Read the model definition and answer for the solid it produces. Units are mm, in the model's axes. Face numbers are marked on the shaded views. Give positions to 0.01 mm unless a question says otherwise; leave off trailing zeros. Order: outer loops, then holes, each group sorted by start corner. A loop starts at its lowest first (then second) coordinate and runs counter-clockwise, first axis right, second up. Notation, with made-up numbers: (60, -40) - (106, -40) arc R14 ccw to (106, -28) - close; hole circle Ø2 at (-27.75, -14). An arc over 180 degrees is marked (long way). Write each question's results on one line, items separated by ' | '.
from build123d import *

# Parameters (mm, degrees)
SKETCH1_W             = 7
SKETCH1_H             = 12
BOSS_EXTRUDE1_DEPTH   = 5
SKETCH1_W_2           = 8.5
BOSS_EXTRUDE1_2_DEPTH = 5
SKETCH3_W             = 122.5
SKETCH3_H             = 12
BOSS_EXTRUDE2_DEPTH   = 3
SKETCH4_R             = 1.4
CUT_EXTRUDE1_DEPTH    = 3
FILLET1_R             = 3


with BuildPart() as part:
    # Sketch1 → Boss-Extrude1 (new body)
    with BuildSketch(Plane(origin=(0, 0, 0), x_dir=(0, 0, -1), z_dir=(1, 0, 0))):
        with Locations((-57, 0)):
            Rectangle(SKETCH1_W, SKETCH1_H)
    extrude(amount=BOSS_EXTRUDE1_DEPTH)



with BuildPart() as body_2:
    # Sketch1 → Boss-Extrude1 2 (new body)
    with BuildSketch(Plane(origin=(0, 0, 0), x_dir=(0, 0, -1), z_dir=(1, 0, 0))):
        with Locations((57.75, 0)):
            Rectangle(SKETCH1_W_2, SKETCH1_H)
    extrude(amount=BOSS_EXTRUDE1_2_DEPTH)


with BuildPart() as part_1:
    add(part.part)

    add(body_2.part)  # Boss-Extrude2 merges body 2
    # Sketch3 → Boss-Extrude2 (add)
    with BuildSketch(Plane(origin=(5, 0, 0), x_dir=(0, 0, -1), z_dir=(1, 0, 0))):
        with Locations((0.75, 0)):
            Rectangle(SKETCH3_W, SKETCH3_H)
    extrude(amount=BOSS_EXTRUDE2_DEPTH)

    # Sketch4 → Cut-Extrude1 (cut)
    with BuildSketch(Plane(origin=(8, 0, 0), x_dir=(0, 0, -1), z_dir=(1, 0, 0))):
        with BuildLine():
            Line((-19.25, 4.4), (-29.25, 4.4))
            ThreePointArc((-29.25, 4.4), (-30.65, 3), (-29.25, 1.6))
            Line((-29.25, 1.6), (-19.25, 1.6))
            ThreePointArc((-19.25, 1.6), (-20.65, 3), (-19.25, 4.4))
        make_face()
        with Locations((-19.25, 3)):
            Circle(SKETCH4_R)
        with BuildLine():
            Line((-9.25, 4.4), (-19.25, 4.4))
            ThreePointArc((-19.25, 4.4), (-18.260050506, 3.989949494), (-17.85, 3))
            ThreePointArc((-17.85, 3), (-18.260050506, 2.010050506), (-19.25, 1.6))
            Line((-19.25, 1.6), (-9.25, 1.6))
            ThreePointArc((-9.25, 1.6), (-7.85, 3), (-9.25, 4.4))
        make_face()
        with BuildLine():
            Line((-9.25, -1.6), (-19.250000006, -1.6))
            ThreePointArc((-19.250000006, -1.6), (-18.260050509, -2.010050504), (-17.85, -3))
            ThreePointArc((-17.85, -3), (-18.260050506, -3.989949494), (-19.25, -4.4))
            Line((-19.25, -4.4), (-9.25, -4.4))
            ThreePointArc((-9.25, -4.4), (-7.85, -3), (-9.25, -1.6))
        make_face()
        with Locations((-19.25, -3)):
            Circle(SKETCH4_R)
        with BuildLine():
            Line((-19.250000006, -1.6), (-29.25, -1.6))
            ThreePointArc((-29.25, -1.6), (-30.65, -3), (-29.25, -4.4))
            Line((-29.25, -4.4), (-19.25, -4.4))
            ThreePointArc((-19.25, -4.4), (-20.65, -3.000000003), (-19.250000006, -1.6))
        make_face()
        with BuildLine():
            Line((10.75, -4.4), (20.75, -4.4))
            ThreePointArc((20.75, -4.4), (19.35, -3), (20.75, -1.6))
            Line((20.75, -1.6), (10.75, -1.6))
            ThreePointArc((10.75, -1.6), (9.35, -3), (10.75, -4.4))
        make_face()
        with BuildLine():
            Line((10.75, 1.6), (20.75, 1.6))
            ThreePointArc((20.75, 1.6), (19.35, 2.999999987), (20.749999974, 4.4))
            Line((20.749999974, 4.4), (10.75, 4.4))
            ThreePointArc((10.75, 4.4), (9.35, 3), (10.75, 1.6))
        make_face()
        with Locations((20.75, 3)):
            Circle(SKETCH4_R)
        with BuildLine():
            Line((20.75, 1.6), (30.75, 1.6))
            ThreePointArc((30.75, 1.6), (32.15, 3), (30.75, 4.4))
            Line((30.75, 4.4), (20.749999974, 4.4))
            ThreePointArc((20.749999974, 4.4), (21.739949484, 3.989949503), (22.15, 3))
            ThreePointArc((22.15, 3), (21.739949494, 2.010050506), (20.75, 1.6))
        make_face()
        with BuildLine():
            Line((20.75, -4.4), (30.75, -4.4))
            ThreePointArc((30.75, -4.4), (32.15, -3), (30.75, -1.6))
            Line((30.75, -1.6), (20.75, -1.6))
            ThreePointArc((20.75, -1.6), (21.739949494, -2.010050506), (22.15, -3))
            ThreePointArc((22.15, -3), (21.739949494, -3.989949494), (20.75, -4.4))
        make_face()
        with Locations((20.75, -3)):
            Circle(SKETCH4_R)
    extrude(amount=-CUT_EXTRUDE1_DEPTH, mode=Mode.SUBTRACT)

    # Fillet1
    fillet1_edges = [part_1.edges().sort_by_distance(p)[0] for p in [
        (8, 0, 60.5),
        (8, 0, -62),
    ]]
    fillet(fillet1_edges, radius=FILLET1_R)


solid = part_1.part
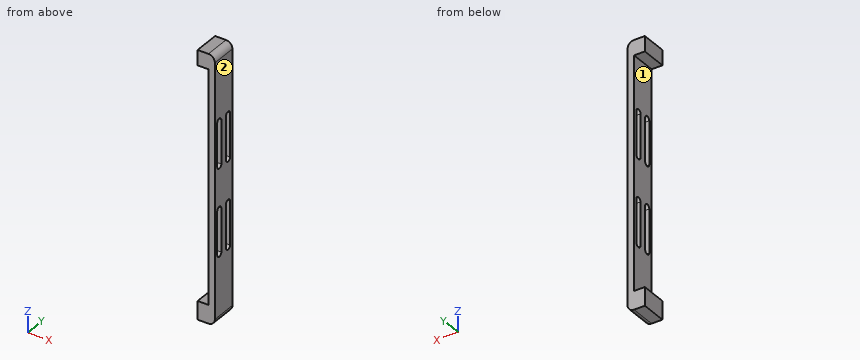
(1) Consider probe 1 along Y at (x, z) = (6.5, 17.5); probe 2 along Z at (x, y) = (4.5, 1.5); probe 3 along X at (y, z) = (-1, -37.5). Determine where each line is inside the solid, lowest interval first. Write a range as [from, to].
Conclusion:
probe 1: [-6, -4.4], [-1.6, 1.6], [4.4, 6] | probe 2: [-62, -53.5], [53.5, 60.5] | probe 3: [5, 8]
(2) Each of these flat-tipped pins is pushed along its axis until it touches: pin 1 (1.5 mm diameter, centred on x = 6.5, y = 3.5, fed in from -Z); pin 2 (1.5 mm diameter, centred on y = 2, z = 3.5, fed in from -X). Where does it stop, or does it pass through?
Conclusion:
pin 1: z = -61.9 | pin 2: x = 5
(3) Section A-A (x = 1.25) is taken. Give the vertices of the cut face in (y, z).
Conclusion:
outline: (-6, -62) - (6, -62) - (6, -53.5) - (-6, -53.5) - close; (-6, 53.5) - (6, 53.5) - (6, 60.5) - (-6, 60.5) - close
(4) Section C-C (z = 26) is taken. Give the vertices of the cut face in (x, y).
Conclusion:
outline: (5, -6) - (8, -6) - (8, -4.4) - (5, -4.4) - close; (5, -1.6) - (8, -1.6) - (8, 1.6) - (5, 1.6) - close; (5, 4.4) - (8, 4.4) - (8, 6) - (5, 6) - close
(5) The mould has two halves that part along Z. Classify the marked faces 1 and 2: pulls with the +Z half, pulls with the -Z half, needs draft (parallel to the pull), parting line crosses it, or undercut.
Conclusion:
face 1: undercut | face 2: needs draft
(6) Section D-D (z = 41) is taken. Give the vertices of the cut face in (x, y), plus the area to 3 significant figures.
Conclusion:
outline: (5, -6) - (8, -6) - (8, 6) - (5, 6) - close | area: 36.0 mm^2
(7) Section B-B (y = -3) is taken. Give the vertices of the cut face in (x, z), plus the area to 3 significant figures.
Conclusion:
outline: (0, -62) - (5, -62) arc R3 ccw to (8, -59) - (8, -32.15) - (5, -32.15) - (5, -53.5) - (0, -53.5) - close; (0, 53.5) - (5, 53.5) - (5, 30.65) - (8, 30.65) - (8, 57.5) arc R3 ccw to (5, 60.5) - (0, 60.5) - close; (5, -9.35) - (8, -9.35) - (8, 7.85) - (5, 7.85) - close | area: 304 mm^2
